```python
from build123d import *

# Parameters (mm, degrees)
SKETCH1_R                      = 4.95
SKETCH1_R_2                    = 4.45
BOSS_EXTRUDE1_DEPTH            = 47.6
SKETCH5_R                      = 7.7
SKETCH5_R_2                    = 4.45
BOSS_EXTRUDE3_DEPTH            = 2
SKETCH2_R                      = 0.625
CUT_EXTRUDE1_DEPTH             = 0.7
CUT_EXTRUDE1_DIRECTION_2_REACH = 4


with BuildPart() as part:
    # Sketch1 → Boss-Extrude1 (new body)
    with BuildSketch(Plane.XY):
        Circle(SKETCH1_R)
        Circle(SKETCH1_R_2, mode=Mode.SUBTRACT)
    extrude(amount=BOSS_EXTRUDE1_DEPTH)

    # Sketch5 → Boss-Extrude3 (add)
    with BuildSketch(Plane.XY.offset(47.6)):
        Circle(SKETCH5_R)
        Circle(SKETCH5_R_2, mode=Mode.SUBTRACT)
    extrude(amount=BOSS_EXTRUDE3_DEPTH)

    # Sketch2 → Cut-Extrude1 (cut)
    with BuildSketch(Plane(origin=(0, 0, 47.6), x_dir=(-1, 0, 0), z_dir=(0, 0, -1))):
        with Locations((0, 4.45)):
            Circle(SKETCH2_R)
        with Locations((1.375125625, 4.232201498)):
            Circle(SKETCH2_R)
    extrude(amount=CUT_EXTRUDE1_DEPTH, mode=Mode.SUBTRACT)

    # Sketch2 → Cut-Extrude1 direction 2 (cut, up to next)
    with BuildSketch(Plane(origin=(0, 0, 47.6), x_dir=(-1, 0, 0), z_dir=(0, 0, -1)), mode=Mode.PRIVATE) as cut_extrude1_direction_2_sk1:
        with Locations((0, 4.45)):
            Circle(SKETCH2_R)
    cut_extrude1_direction_2_tool1 = extrude(cut_extrude1_direction_2_sk1.sketch, amount=-CUT_EXTRUDE1_DIRECTION_2_REACH, mode=Mode.PRIVATE) & part.part
    add(cut_extrude1_direction_2_tool1.solids().sort_by_distance((0, 4.45, 47.6))[0], mode=Mode.SUBTRACT)
    # Sketch2 → Cut-Extrude1 direction 2 (cut, up to next)
    with BuildSketch(Plane(origin=(0, 0, 47.6), x_dir=(-1, 0, 0), z_dir=(0, 0, -1)), mode=Mode.PRIVATE) as cut_extrude1_direction_2_sk2:
        with Locations((1.375125625, 4.232201498)):
            Circle(SKETCH2_R)
    cut_extrude1_direction_2_tool2 = extrude(cut_extrude1_direction_2_sk2.sketch, amount=-CUT_EXTRUDE1_DIRECTION_2_REACH, mode=Mode.PRIVATE) & part.part
    add(cut_extrude1_direction_2_tool2.solids().sort_by_distance((-1.375126, 4.232201, 47.6))[0], mode=Mode.SUBTRACT)


solid = part.part
```
Input: part model. Units: mm. Frame: model coordinates. A direction names the side the tool comes from. Give positions to 0.01 mm unless a question says otherwise; leave off trailing zeros. Order: outer loops, then holes, each group sorted by start corner. A loop starts at its lowest first (then second) coordinate and runs counter-clockwise, first axis right, second up. Notation, with made-up numbers: M -8.5,5 L 35.5,5 A33 cw 35.5,34 Z; hole C 55,42 d5. An arc over 180 degrees is marked long. Return JSON: item names as keys, results as strings.
Item 1: Cut plane B-B (x = 1.25). Return loops of the section in (y, z).
Solutions:
{"outline": "M -7.6,47.6 L -4.79,47.6 L -4.79,0 L -4.27,0 L -4.27,49.6 L -7.6,49.6 Z; M 4.27,0 L 4.79,0 L 4.79,47.6 L 7.6,47.6 L 7.6,49.6 L 4.27,49.6 Z"}
Item 2: Access query for faces 1 (the flat face through (-1.4, 4.4, 46.9)), 2 (the cylindrical face through (4.72, 1.49, 23.47)). Directions: +Z, -Z, +X, -X, +Y, -Y. A direction counts if a zero-diameter tool reaches every point of the face in a straight line with its end or side. Return the directions, or none.
Solutions:
{"face 1": "+Z", "face 2": "-Z"}
Item 3: Cut plane A-A (y = 0). Return loops of the section in (x, z), then the cut area to 3 significant figures.
Solutions:
{"outline": "M -7.7,47.6 L -4.95,47.6 L -4.95,0 L -4.45,0 L -4.45,49.6 L -7.7,49.6 Z; M 4.45,0 L 4.95,0 L 4.95,47.6 L 7.7,47.6 L 7.7,49.6 L 4.45,49.6 Z", "area": "60.6 mm^2"}
Item 4: First-contact query: P1, Ø1.5, axis at y = 0.5, z = 19, coming from the +X side; P2, Ø5.5, axis at x = 0, y = 0, coming from the +Z side; P3, Ø8, axis at x = -1.5, y = -3, coming from the -Z side; P4, Ø4, axis at x = -2.5, z = 27, coming from the -Y side. Flat tips, straight axial feed; report the tip coordinate or a pass-through.
Solutions:
{"P1": "x = 4.95", "P2": "through", "P3": "z = 0", "P4": "y = -4.92"}
Item 5: Cut plane C-C (z = 42). Return loops of the section in (x, y).
Solutions:
{"outline": "C 0,0 d9.9; hole C 0,0 d8.9"}
Item 6: Cut plane D-D (x = 6.5). Return loops of the section in (y, z).
Solutions:
{"outline": "M -4.13,47.6 L 4.13,47.6 L 4.13,49.6 L -4.13,49.6 Z"}
Item 7: Ray query, probe 1 along X at (y, z) = (0, 36); probe 2 along Y at (x, z) = (-2.5, 4). Return the intervals inside material, ascending.
Solutions:
{"probe 1": "-4.95 to -4.45, 4.45 to 4.95", "probe 2": "-4.27 to -3.68, 3.68 to 4.27"}
Item 8: Pull-direction query (X, two-part tool) for faces 3 (the cylindrical face through (-1.669, -7.517, 48.586)), 4 (the cylindrical face through (-0.965, -4.344, 24.453)), 5 (the flat face through (3.3, -3.3, 49.6)); classes: +X half, -X half, draft (parallel to the pull), parting line (faces both ways), or undercut.
Solutions:
{"face 3": "parting line", "face 4": "undercut", "face 5": "draft"}
